Build history of the part. All positions in model axes, mm. A direction names the side the tool comes from. Round coordinates to 2 decimals unless told otherwise and drop trailing zeros. Write each loop counter-clockwise with the first axis right and the second up, starting at its lowest first coordinate (ties: lowest second). Pieces come first, ordered by that corner, then holes.
from build123d import *

# Parameters (mm, degrees)
SKETCH_3_R               = 7.5
EXTRUDE_2_DEPTH          = 3
CUT_EXTRUDE_1_DEPTH      = 5
SKETCH_5_R               = 1
CUT_EXTRUDE_2_DEPTH      = 5
PATTERN_CIRCULAR_1_COUNT = 6
CUT_EXTRUDE_3_DEPTH      = 10


with BuildPart() as part:
    # 스케치3 → 보스-돌출2 (new body)
    with BuildSketch(Plane(origin=(0, 0, 0), x_dir=(1, 0, 0), z_dir=(0, 1, 0))):
        with Locations(Location((0, 0, 0), (0, 0, 270))):
            Circle(SKETCH_3_R)
    extrude(amount=EXTRUDE_2_DEPTH)

    # 스케치4 → 컷-돌출1 (cut)
    with BuildSketch(Plane(origin=(0, 3, 0), x_dir=(1, 0, 0), z_dir=(0, 1, 0))):
        Polygon((4.05, 2.33826859), (0, 4.67653718), (-4.05, 2.33826859), (-4.05, -2.33826859), (0, -4.67653718), (4.05, -2.33826859), align=None)
    extrude(amount=-CUT_EXTRUDE_1_DEPTH, mode=Mode.SUBTRACT)

    # 스케치5 → 컷-돌출2 (cut)
    with BuildSketch(Plane(origin=(0, 3, 0), x_dir=(1, 0, 0), z_dir=(0, 1, 0))):
        with Locations((0, 3.67653718)):
            Circle(SKETCH_5_R)
    cut_extrude_2 = extrude(amount=-CUT_EXTRUDE_2_DEPTH, mode=Mode.SUBTRACT)

    # 원형 패턴1: 컷-돌출2 ×6 about axis
    pattern_circular_1_axis = Axis((0, 0, 0), (0, 1, 0))
    for i in range(1, PATTERN_CIRCULAR_1_COUNT):
        add(cut_extrude_2.rotate(pattern_circular_1_axis, i * 360 / PATTERN_CIRCULAR_1_COUNT), mode=Mode.SUBTRACT)

    # 스케치6 → 컷-돌출3 (cut)
    with BuildSketch(Plane(origin=(0, 3, 0), x_dir=(1, 0, 0), z_dir=(0, 1, 0))):
        with BuildLine():
            Line((-2.5, -8.065496872), (-2.5, -2.774670645))
            ThreePointArc((-2.5, -2.774670645), (0, -0.274670645), (2.5, -2.774670645))
            Line((2.5, -2.774670645), (2.5, -8.065496872))
            ThreePointArc((2.5, -8.065496872), (0, -10.565496872), (-2.5, -8.065496872))
        make_face()
    extrude(amount=-CUT_EXTRUDE_3_DEPTH, mode=Mode.SUBTRACT)


solid = part.part
1) Slice it at D-D (x = 0). Write the cut outline in (y, z).
Results:
outline: (0, -7.5) - (3, -7.5) - (3, -4.68) - (0, -4.68) - close
2) Slice it at A-A (z = 0). Write the cut outline in (x, y), plus the area to 3 significant figures.
Results:
outline: (-7.5, 0) - (-4.05, 0) - (-4.05, 3) - (-7.5, 3) - close; (4.05, 0) - (7.5, 0) - (7.5, 3) - (4.05, 3) - close
area: 20.7 mm2
3) Slice it at C-C (y = 1). Write the cut outline in (x, z).
Results:
outline: (-4.05, -1.34) - (-4.05, 1.34) arc R1 cw to (-3.18, 2.84) - (-2.5, 3.23) - (-2.5, 7.07) arc R7.5 ccw (long way) to (2.5, 7.07) - (2.5, 3.23) - (3.18, 2.84) arc R1 cw to (4.05, 1.34) - (4.05, -1.34) arc R1 cw to (3.18, -2.84) - (0.87, -4.18) arc R1 cw to (-0.87, -4.18) - (-3.18, -2.84) arc R1 cw to start
4) Slice it at B-B (x = -3). Write the cut outline in (y, z).
Results:
outline: (0, -6.87) - (3, -6.87) - (3, -2.94) - (0, -2.94) - close; (0, 2.94) - (3, 2.94) - (3, 6.87) - (0, 6.87) - close
5) Mould opens along X. For faces 1 (the cylindrical face through (0.294, 1.479, -7.494)), 2 (the flat face through (2.04, 1.52, -3.5)), 3 (the flat face through (-3, 3, -4)), 4 (the cylindrical face through (-4.057, 1.521, 2.326)) say: released by +X, released by -X, zero draft, split by the parting line, or undercut.
Results:
face 1: split by the parting line
face 2: undercut
face 3: zero draft
face 4: undercut
6) Which spindle directions (+Z, -Z, +X, -X, +Y, -Y) get a long thin tool onto all of the face, cutting with end or side? Do faces 5 (the flat face through (-2.5, 2, 5)), 6 (the flat face through (-3, 0, -4)), 7 (the flat face through (-4.05, 2, 0)). Say none if no direction does.
Results:
face 5: +Z, +Y, -Y
face 6: +Z, -Z, +X, -X, -Y
face 7: +Y, -Y
7) Wall check: L1, parallel to X at y = 2.3, z = 0; L2, parallel to Z at x = -3.75, y = 2.15; L3, parallel to X at y = 1.5, z = 5.25. Give the ranges that are in metal, low to high.
Results:
L1: x = -7.5 to -4.05, 4.05 to 7.5
L2: z = -6.5 to -2.66, 2.66 to 6.5
L3: x = -5.36 to -2.5, 2.5 to 5.36
8) Pin check, flat tip, straight feed: pin 1 Ø1.5 at (y, z) = (1, -5.5) entering from -X. Stop position of the tip, or through.
Results:
pin 1: stops at x = -5.8
